Source: CAD feature listing. Evaluate the final solid. Frame: model axes, mm. Round coordinates to 2 decimals unless told otherwise and drop trailing zeros. Write each loop counter-clockwise with the first axis right and the second up, starting at its lowest first coordinate (ties: lowest second). Pieces come first, ordered by that corner, then holes.
from build123d import *

# Parameters (mm, degrees)
ESBO_O1_R                = 2.998945894
ESBO_O1_R_2              = 1.5
RESSALTO_EXTRUS_O1_DEPTH = 2
ESBO_O3_W                = 77.000000909
ESBO_O3_H                = 20.799996635
CORTE_EXTRUS_O2_DEPTH    = 3


with BuildPart() as part:
    # Esboço1 → Ressalto-extrusão1 (new body)
    with BuildSketch(Plane.XY):
        with BuildLine():
            Line((-0.452, 5.715), (-25.598, 67.691))
            ThreePointArc((-25.598, 67.691), (-27.830124117, 70.420084628), (-31.186, 71.501))
            Line((-31.186, 71.501), (-127.706, 71.501))
            ThreePointArc((-127.706, 71.501), (-130.895769937, 70.507154905), (-133.04, 67.945))
            Line((-133.04, 67.945), (-159.456, 5.461))
            ThreePointArc((-159.456, 5.461), (-159.249042624, 1.900068852), (-156.154, 0.127))
            Line((-156.154, 0.127), (-119.832, 0.127))
            ThreePointArc((-119.832, 0.127), (-116.845272565, 0.798888491), (-114.244, 2.413))
            Line((-114.244, 2.413), (-103.576, 13.081))
            ThreePointArc((-103.576, 13.081), (-100.992547951, 14.814205491), (-97.988, 15.621))
            Line((-97.988, 15.621), (-62.174, 15.621))
            ThreePointArc((-62.174, 15.621), (-59.187272565, 14.949111509), (-56.586, 13.335))
            Line((-56.586, 13.335), (-45.918, 2.667))
            ThreePointArc((-45.918, 2.667), (-43.605600005, 0.941799989), (-40.838, 0.127))
            Line((-40.838, 0.127), (-3.754, 0.127))
            ThreePointArc((-3.754, 0.127), (-0.686880545, 2.08420214), (-0.452, 5.715))
        make_face()
        with Locations((-127.610794879, 65.579692319)):
            Circle(ESBO_O1_R, mode=Mode.SUBTRACT)
        with Locations((-105.664, 67.501)):
            Circle(ESBO_O1_R_2, mode=Mode.SUBTRACT)
        with Locations((-79.5, 67.501)):
            Circle(ESBO_O1_R_2, mode=Mode.SUBTRACT)
        with Locations((-4, 4)):
            Circle(ESBO_O1_R_2, mode=Mode.SUBTRACT)
        with Locations((-155.893, 4)):
            Circle(ESBO_O1_R_2, mode=Mode.SUBTRACT)
    extrude(amount=RESSALTO_EXTRUS_O1_DEPTH)

    # Esboço3 → Corte-extrusão2 (cut, through all)
    with BuildSketch(Plane(origin=(0, 0, 0), x_dir=(-1, 0, 0), z_dir=(0, 0, -1))):
        with Locations((79.512001037, 51.64081955)):
            Rectangle(ESBO_O3_W, ESBO_O3_H)
    extrude(amount=-CORTE_EXTRUS_O2_DEPTH, mode=Mode.SUBTRACT)


solid = part.part
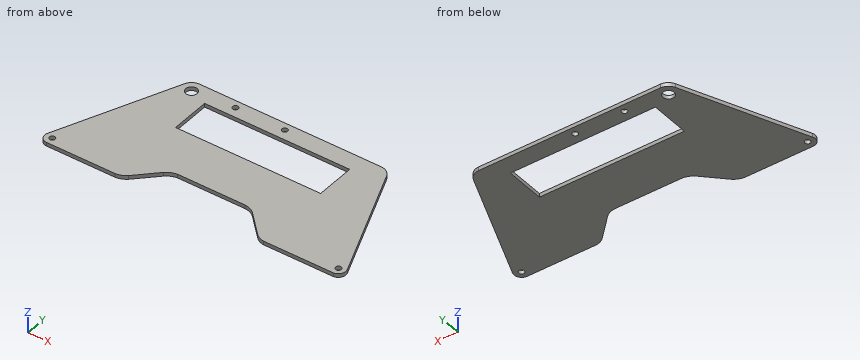
1) Section query C-C on z = 1.55. Return the cut outline in (x, y) (3 decimals), then the cut area to 3 significant figures.
Taken from the geometry:
outline: (-159.456, 5.461) arc R3.746 ccw to (-156.154, 0.127) - (-119.832, 0.127) arc R9.206 ccw to (-114.244, 2.413) - (-103.576, 13.081) arc R9.511 cw to (-97.988, 15.621) - (-62.174, 15.621) arc R9.206 cw to (-56.586, 13.335) - (-45.918, 2.667) arc R8.177 ccw to (-40.838, 0.127) - (-3.754, 0.127) arc R4.024 ccw to (-0.452, 5.715) - (-25.598, 67.691) arc R6.231 ccw to (-31.186, 71.501) - (-127.706, 71.501) arc R5.922 ccw to (-133.04, 67.945) - close; hole circle Ø3 at (-155.893, 4); hole circle Ø5.998 at (-127.611, 65.58); hole (-118.012, 41.241) - (-41.012, 41.241) - (-41.012, 62.041) - (-118.012, 62.041) - close; hole circle Ø3 at (-105.664, 67.501); hole circle Ø3 at (-79.5, 67.501); hole circle Ø3 at (-4, 4)
area: 6,990 mm2
2) Contact query for flat-ended pins moving along their axis: P1, Ø1.8, axis at x = -105.664, y = 67.501, coming from the -Z side; P2, Ø1, axis at x = -63, z = 0.5, coming from the -Y side. Output: stop coordinate, or through.
Taken from the geometry:
P1: passes through
P2: stops at y = 15.62
3) Section query D-D on x = -146.5. Return the cut outline in (y, z), then the cut area to 3 significant figures.
Taken from the geometry:
outline: (0.13, 0) - (36.11, 0) - (36.11, 2) - (0.13, 2) - close
area: 72.0 mm2
4) Section query A-A on x = -68. Return the cut outline in (y, z).
Taken from the geometry:
outline: (15.62, 0) - (41.24, 0) - (41.24, 2) - (15.62, 2) - close; (62.04, 0) - (71.5, 0) - (71.5, 2) - (62.04, 2) - close
5) Material intervals for line 1 (Y direction, x = -79.5, z = 1); line 2 (Y direction, x = -84.5, z = 0.8); line 3 (X direction, y = 67, z = 0.15), sorted ascending.
Taken from the geometry:
line 1: y = 15.62 to 41.24, 62.04 to 66, 69 to 71.5
line 2: y = 15.62 to 41.24, 62.04 to 71.5
line 3: x = -133.44 to -130.25, -124.97 to -107.08, -104.25 to -80.91, -78.09 to -25.32
6) Section query B-B on y = 49.5. Return the cut outline in (x, z).
Taken from the geometry:
outline: (-140.84, 0) - (-118.01, 0) - (-118.01, 2) - (-140.84, 2) - close; (-41.01, 0) - (-18.22, 0) - (-18.22, 2) - (-41.01, 2) - close
